For this review, take the finished solid that the model builds, in its own axes (mm). A direction names the side the tool comes from. Round coordinates to 2 decimals unless told otherwise and drop trailing zeros. Order: outer loops, then holes, each group sorted by start corner. A loop starts at its lowest first (then second) coordinate and runs counter-clockwise, first axis right, second up. Notation, with made-up numbers: M 57.5,87.25 L 68.5,87.25 A33 ccw 68.5,121.25 Z; hole C -21.75,-32.75 d7. An arc over 180 degrees is marked long. Answer as a JSON object with one key per item and string values.
from build123d import *

# Parameters (mm, degrees)
F1_DEPTH = 2.8
F2_R     = 3
F3_R     = 1


with BuildPart() as f1:
    # F0 (on Top) → F1 (new body)
    with BuildSketch(Plane.XY):
        with BuildLine():
            ThreePointArc((7.5, -12.3924725737), (12.6186961846, -7.1127971356), (14.4852813742, 0))
            ThreePointArc((14.4852813742, 0), (13.869819685, 4.1774966664), (12.075735029, 8))
            Line((12.075735029, 8), (6, 8))
            Line((6, 8), (6, 6))
            Line((6, 6), (6, -6))
            Line((6, -6), (-6, -6))
            Line((-6, -6), (-6, 6))
            Line((-6, 6), (-6, 8))
            Line((-6, 8), (-12.075735029, 8))
            ThreePointArc((-12.075735029, 8), (-14.1338453684, -3.1714021492), (-7.5, -12.3924725737))
            Line((-7.5, -12.3924725737), (7.5, -12.3924725737))
        make_face()
        with BuildLine():
            Line((7.5, -36.3924725737), (7.5, -12.3924725737))
            ThreePointArc((7.5, -12.3924725737), (0, -14.4852813742), (-7.5, -12.3924725737))
            Line((-7.5, -12.3924725737), (-7.5, -21.3924725737))
            ThreePointArc((-7.5, -21.3924725737), (-1.5, -28.8924725737), (-7.5, -36.3924725737))
            Line((-7.5, -36.3924725737), (7.5, -36.3924725737))
        make_face()
        with BuildLine():
            ThreePointArc((-7.5, -12.3924725737), (0, -14.4852813742), (7.5, -12.3924725737))
            Line((7.5, -12.3924725737), (-7.5, -12.3924725737))
        make_face()
    extrude(amount=F1_DEPTH)

    # F2
    f2_edges = [f1.edges().sort_by_distance(p)[0] for p in [
        (-7.5, -12.392473, 1.4),
        (7.5, -12.392473, 1.4),
        (6, -6, 1.4),
        (-6, -6, 1.4),
    ]]
    fillet(f2_edges, radius=F2_R)

    # F3
    f3_edges = [f1.edges().sort_by_distance(p)[0] for p in [
        (-7.5, -36.392473, 1.4),
        (7.5, -36.392473, 1.4),
        (6, 8, 1.4),
        (-6, 8, 1.4),
        (-12.075735, 8, 1.4),
        (12.075735, 8, 1.4),
        (-7.5, -21.392473, 1.4),
    ]]
    fillet(f3_edges, radius=F3_R)


solid = f1.part
1) Add section B-B on x = -2.25. State the section outline as (y, z) points, and give its area (3 significant figures).
Geometry check:
{"outline": "M -36.39,0 L -32.2,0 L -32.2,2.8 L -36.39,2.8 Z; M -25.58,0 L -6,0 L -6,2.8 L -25.58,2.8 Z", "area": "66.6 mm²"}
2) Mouldability with a two-part tool opening along Y and no side actions: class faces 5 (the cylindrical face through (-4.352, -35.763, 1.42)), 6 (the cylindrical face through (7.215, -36.092, 1.42)), 7 (the cylindrical face through (-6.285, 7.699, 1.42)) as +Y half, -Y half, draft (parallel to the pull), parting line (faces both ways), or undercut.
Geometry check:
{"face 5": "undercut", "face 6": "-Y half", "face 7": "+Y half"}
3) Machinability: for faces 1 (the flat face through (-7.5, -17, 1)), 2 (the flat face through (7.5, -25, 1)), 3 (the flat face through (1, -36.392, 1)), 4 (the flat face through (6, 2, 1)), which of the approach directions +Z, -Z, +X, -X, +Y, -Y give a long, thin tool a straight path to every point of the face, cutting with its end or side? Answer none if there is none.
Geometry check:
{"face 1": "+Z, -Z, -X, -Y", "face 2": "+Z, -Z, +X, -Y", "face 3": "+Z, -Z, +X, -X, -Y", "face 4": "+Z, -Z, +Y"}
4) Add section C-C on z = 2.35. State the section outline as (x, y) points (1 decimal), and give its area (3 significant figures).
Geometry check:
{"outline": "M -12.4,7.5 A14.5 ccw -8.7,-11.6 A3 cw -7.5,-14 L -7.5,-20.6 A1 ccw -6.8,-21.6 A7.7 cw -4.1,-34.6 A1 ccw -3.4,-36.4 L 6.5,-36.4 A1 ccw 7.5,-35.4 L 7.5,-14 A3 cw 8.7,-11.6 A14.5 ccw 12.4,7.5 A1 ccw 11.5,8 L 7,8 A1 ccw 6,7 L 6,-3 A3 cw 3,-6 L -3,-6 A3 cw -6,-3 L -6,7 A1 ccw -7,8 L -11.5,8 A1 ccw Z", "area": "654 mm²"}
5) For L1, parallel to X at y = -17.5, z = 1.95; L2, parallel to X at y = -4.5, z = 2.2; L3, parallel to X at y = -3, z = 1.8, list the stretches that pass through material, from the lowest coordinate up.
Geometry check:
{"L1": "x = -7.5 to 7.5", "L2": "x = -13.77 to -5.6, 5.6 to 13.77", "L3": "x = -14.17 to -6, 6 to 14.17"}
6) Insertion check: P1, Ø1, axis at y = -17, z = 2, coming from the -X side; P2, Ø1.5, axis at y = -26, z = 2, coming from the +X side; P3, Ø1.4, axis at y = 0.5, z = 1, coming from the +X side. Each pin has a flat end and moves straight along its axis. Give the tip position at first contact, or say it passes through.
Geometry check:
{"P1": "stops at x = -7.5", "P2": "stops at x = 7.5", "P3": "stops at x = 14.49"}
7) Add section A-A on y = 4. State the section outline as (x, z) points.
Geometry check:
{"outline": "M -13.92,0 L -6,0 L -6,2.8 L -13.92,2.8 Z; M 6,0 L 13.92,0 L 13.92,2.8 L 6,2.8 Z"}
8) Add section D-D on y = -19.5. State the section outline as (x, z) points.
Geometry check:
{"outline": "M -7.5,0 L 7.5,0 L 7.5,2.8 L -7.5,2.8 Z"}
